from build123d import *

# Parameters (mm, degrees)
SKETCH1_W           = 300
SKETCH1_H           = 180
SKETCH1_R           = 15.290295186
BOSS_EXTRUDE1_DEPTH = 10
SKETCH2_W           = 25
SKETCH2_H           = 3.625381299
SKETCH2_W_2         = 20
SKETCH2_H_2         = 4.172919767
BOSS_EXTRUDE2_DEPTH = 27
SKETCH3_W           = 119.797948109
SKETCH3_H           = 135
BOSS_EXTRUDE3_DEPTH = 5


with BuildPart() as part:
    # Sketch1 → Boss-Extrude1 (new body)
    with BuildSketch(Plane.XY):
        with Locations((50.602409639, -56.56626506)):
            Rectangle(SKETCH1_W, SKETCH1_H)
        with Locations((161.4744217, -60.89830155)):
            Circle(SKETCH1_R, mode=Mode.SUBTRACT)
    extrude(amount=BOSS_EXTRUDE1_DEPTH)

    # Sketch2 → Boss-Extrude2 (add)
    with BuildSketch(Plane.XY.offset(10)):
        Polygon((-61.566986646, 8.214667576), (-61.566986646, -116.785332424), (-61.566986646, -121.785332424), (20.433013354, -121.785332424), (20.433013354, -116.785332424), (-56.566986646, -116.785332424), (-56.566986646, 8.214667576), (-16.566986646, 8.214667576), (-16.566986646, 13.214667576), (-56.566986646, 13.214667576), (-61.566986646, 13.214667576), align=None)
        with Locations((45.914281805, 11.395862513)):
            Rectangle(SKETCH2_W, SKETCH2_H)
        with Locations((48.230961463, -119.698872541)):
            Rectangle(SKETCH2_W_2, SKETCH2_H_2)
    extrude(amount=BOSS_EXTRUDE2_DEPTH)

    # Sketch3 → Boss-Extrude3 (add)
    with BuildSketch(Plane.XY.offset(37)):
        with Locations((-1.668012591, -54.285332424)):
            Rectangle(SKETCH3_W, SKETCH3_H)
    extrude(amount=BOSS_EXTRUDE3_DEPTH)


solid = part.part
Source: CAD feature listing. Evaluate the final solid. Frame: model axes, mm. A direction names the side the tool comes from. Give positions to 0.01 mm unless a question says otherwise; leave off trailing zeros. Write each loop counter-clockwise with the first axis right and the second up, starting at its lowest first coordinate (ties: lowest second). Pieces come first, ordered by that corner, then holes. Notation, with made-up numbers: M 5.25,23.5 L 18.25,23.5 A21 ccw 18.25,60.5 Z; hole C 89,68 d8. An arc over 180 degrees is marked long. Return JSON: item names as keys, results as strings. Group by question number.
1) Cut plane A-A, the plane z = 14. Output: boundary loops of the cut face in (x, y).
2) Draft query along Z for faces 4 (the face through (49, -146.566, 5)), 5 (the face through (-3, -53, 42)), 6 (the face through (0, -53, 37)). Return one class per face: released by +Z, released by -Z, zero draft, split by the parting line, or undercut.
3) Cut plane C-C, the plane y = -58. Output: boundary loops of the cut face in (x, z).
4) Set-up query: faces 1 (the face through (46, 13.209, 23)), 2 (the face through (-61.567, -55, 26)), 3 (the face through (-37, 8.215, 23)). Return all of +Z, -Z, +X, -X, +Y, -Y with unobstructed straight access to the full face (end or side cutting, diameter ignored); none if empty.
5) First-contact query: pin 1 Ø4 at (y, z) = (-119, 18.5) entering from +X; pin 2 Ø4 at (y, z) = (-29.5, 25) entering from -X; pin 3 Ø8 at (x, y) = (61, -62) entering from -Z; pin 4 Ø12.5 at (x, z) = (48.5, 28.5) entering from -Y. Flat tips, straight axial feed; report the tip coordinate or a pass-through.
6) Cut plane D-D, the plane x = 169.5. Output: boundary loops of the cut face in (y, z), then the cut area to 3 significant figures.
7) Ray query, L1, parallel to X at y = 12.5, z = 30; L2, parallel to Y at x = -53, z = 25; L3, parallel to Y at x = -12.5, z = 24. Return the intervals inside material, ascending.
8) Cut plane B-B, the plane x = -49. Output: boundary loops of the cut face in (y, z), then the cut area to 4 significant figures.
Data:
{
 "1": {"outline": "M -61.57,-121.79 L 20.43,-121.79 L 20.43,-116.79 L -56.57,-116.79 L -56.57,8.21 L -16.57,8.21 L -16.57,13.21 L -61.57,13.21 Z; M 33.41,9.58 L 58.41,9.58 L 58.41,13.21 L 33.41,13.21 Z; M 38.23,-121.79 L 58.23,-121.79 L 58.23,-117.61 L 38.23,-117.61 Z"},
 "2": {"face 4": "zero draft", "face 5": "released by +Z", "face 6": "undercut"},
 "3": {"outline": "M -99.4,0 L 146.46,0 L 146.46,10 L -56.57,10 L -56.57,37 L 58.23,37 L 58.23,42 L -61.57,42 L -61.57,10 L -99.4,10 Z; M 176.49,0 L 200.6,0 L 200.6,10 L 176.49,10 Z"},
 "4": {"face 1": "+Z, +X, -X, +Y", "face 2": "+Z, -X, +Y, -Y", "face 3": "+X"},
 "5": {"pin 1": "stops at x = 58.23", "pin 2": "stops at x = -61.57", "pin 3": "stops at z = 0", "pin 4": "stops at y = -121.79"},
 "6": {"outline": "M -146.57,0 L -73.91,0 L -73.91,10 L -146.57,10 Z; M -47.88,0 L 33.43,0 L 33.43,10 L -47.88,10 Z", "area": "1,540 mm²"},
 "7": {"L1": "x = -61.57 to -16.57, 33.41 to 58.41", "L2": "y = -121.79 to -116.79, 8.21 to 13.21", "L3": "y = -121.79 to -116.79"},
 "8": {"outline": "M -146.57,0 L 33.43,0 L 33.43,10 L 13.21,10 L 13.21,42 L -121.79,42 L -121.79,10 L -146.57,10 Z; hole M -116.79,10 L 8.21,10 L 8.21,37 L -116.79,37 Z", "area": "2,745 mm²"}
}
